Autodesk Inventor part; units mm, degrees
ref_plane "YZ Plane" through (0, 0, 0) normal (1, 0, 0) x (0, 1, 0)
ref_plane "XZ Plane" through (0, 0, 0) normal (0, 1, 0) x (-1, 0, 0)
ref_plane "XY Plane" through (0, 0, 0) normal (0, 0, 1) x (1, 0, 0)
sketch "Sketch1" plane through (0, 0, 0) normal (0, 0, 1) x (1, 0, 0)
  line L0 (5.5, 34.5) -> (27, 34.5)
  line L1 (1.5, 2.5) -> (27, 2.5)
  line L2 (27, 2.5) -> (27, 34.5)
  line L3 (27, 34.5) -> (5.5, 34.5)
  line L4 (1.5, 35.5) -> (1.5, 2.5)
  line L5 (1.5, 76.5) -> (5.5, 76.5)
  line L6 (1.5, 2.5) -> (5.5, 2.5)
  line L7 (5.5, 34.5) -> (5.5, 76.5)
  line L8 (5.5, 76.5) -> (1.5, 76.5)
  line L9 (1.5, 76.5) -> (1.5, 2.5)
  point P0 (0, 0)
  dimension "d0" = 32
  dimension "d2" = 21.5
  dimension "d3" = 42
  dimension "d17" = 4
extrude "Extrusion1" add sketch "Sketch1" along normal blind 1.5
sketch "Sketch2" plane through (0, 0, 0) normal (0, 0, -1) x (-1, 0, 0)
  line L0 (-27, 2.5) -> (-27, 34.5)
  line L1 (-27, 34.5) -> (-5.5, 34.5)
  line L2 (-5.5, 34.5) -> (-5.5, 26.5)
  line L3 (-5.5, 26.5) -> (-27, 26.5)
  line L4 (-27, 26.5) -> (-27, 34.5)
  line L5 (-1.5, 2.5) -> (-27, 2.5)
  line L6 (-27, 2.5) -> (-5.5, 2.5)
  line L7 (-5.5, 2.5) -> (-5.5, 10.5)
  line L8 (-5.5, 10.5) -> (-27, 10.5)
  line L9 (-27, 10.5) -> (-27, 2.5)
  point P0 (0, 0)
  point P1 (-27, 10.5)
  point P2 (-27, 26.5)
  dimension "d6" = 16
extrude "Extrusion2" add sketch "Sketch2" along normal blind 4.5
sketch "Sketch3" plane through (0, 0, 1.5) normal (0, 0, 1) x (1, 0, 0)
  circle A0 centre (8.5, 32.5) radius 1
  circle A1 centre (18.5, 4.5) radius 1
  line L0 (27, 2.5) -> (27, 34.5)
  line L1 (1.5, 2.5) -> (27, 2.5)
  line L2 (27, 34.5) -> (5.5, 34.5)
  point P0 (0, 0)
  dimension "d9" = 2
  dimension "d10" = 2
  dimension "d11" = 18.5
  dimension "d12" = 8.5
  dimension "d13" = 2
  dimension "d14" = 2
extrude "Extrusion3" cut sketch "Sketch3" against normal through all
chamfer "Chamfer1" distance 1.5 angle 45 2 edges at (7.5, 32.5, 1.5) (17.5, 4.5, 1.5)
properties part number "servoholder"
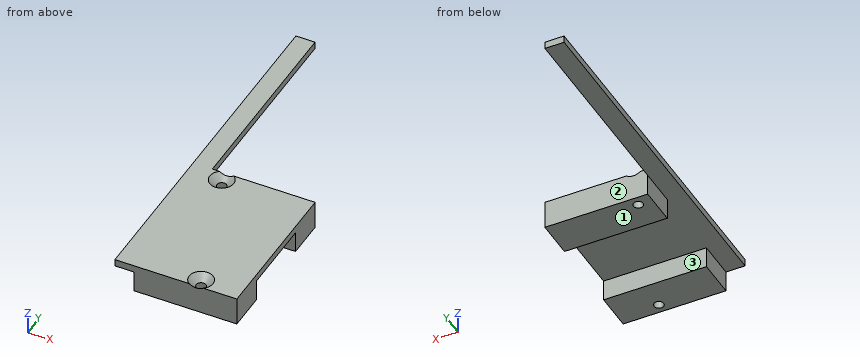
Part model, mm, in its own coordinate system. Face numbers are marked on the shaded views. A direction names the side the tool comes from. Coordinates: 2 decimals unless noted, no trailing zeros. Order: outer loops, then holes, each group sorted by start corner. A loop starts at its lowest first (then second) coordinate and runs counter-clockwise, first axis right, second up.
(1) Slice it at B-B, the plane y = 32.5. Write the cut outline in (x, z), and give its area (3 significant figures).
Check sheet entries:
outline: (1.5, 0) - (5.5, 0) - (5.5, -4.5) - (7.5, -4.5) - (7.5, 0) - (6, 1.5) - (1.5, 1.5) - close; (9.5, -4.5) - (27, -4.5) - (27, 1.5) - (11, 1.5) - (9.5, 0) - close
area: 121 mm2
(2) Slice it at D-D, the plane x = 23.75. Write the cut outline in (y, z), and give its area (3 significant figures).
Check sheet entries:
outline: (2.5, -4.5) - (10.5, -4.5) - (10.5, 0) - (26.5, 0) - (26.5, -4.5) - (34.5, -4.5) - (34.5, 1.5) - (2.5, 1.5) - close
area: 120 mm2
(3) Pin check, flat tips, straight feed: pin 1 Ø1.6 at (y, z) = (65.5, 0.5) entering from +X; pin 2 Ø2 at (x, z) = (15, -0.5) entering from +Y; pin 3 Ø1.6 at (x, y) = (8.5, 32.5) entering from -Z; pin 4 Ø1.3 at (y, z) = (31, -1) entering from -X. Stop position of each tip, or through.
Check sheet entries:
pin 1: stops at x = 5.5
pin 2: stops at y = 34.5
pin 3: passes through
pin 4: stops at x = 5.5
(4) Probe L1, parallel to Y at x = 18.5, z = -3.05; L2, parallel to Y at x = 8.5, z = -3.35; L3, parallel to Y at x = 20.5, z = -3. List the from-to ranges inside material, lowest first.
Check sheet entries:
L1: y = 2.5 to 3.5, 5.5 to 10.5, 26.5 to 34.5
L2: y = 2.5 to 10.5, 26.5 to 31.5, 33.5 to 34.5
L3: y = 2.5 to 10.5, 26.5 to 34.5
(5) Slice it at C-C, the plane x = 18.5. Write the cut outline in (y, z), and give its area (3 significant figures).
Check sheet entries:
outline: (2.5, -4.5) - (3.5, -4.5) - (3.5, 0) - (2.5, 1) - close; (5.5, -4.5) - (10.5, -4.5) - (10.5, 0) - (26.5, 0) - (26.5, -4.5) - (34.5, -4.5) - (34.5, 1.5) - (7, 1.5) - (5.5, 0) - close
area: 106 mm2
(6) Slice it at A-A, the plane z = -2.7. Write the cut outline in (x, y), and give its area (3 significant figures).
Check sheet entries:
outline: (5.5, 2.5) - (27, 2.5) - (27, 10.5) - (5.5, 10.5) - close; (5.5, 26.5) - (27, 26.5) - (27, 34.5) - (5.5, 34.5) - close; hole circle Ø2 at (8.5, 32.5); hole circle Ø2 at (18.5, 4.5)
area: 338 mm2
(7) Tool access for the marked faces 1, 2 and 3: list every direction of +Z, -Z, +X, -X, +Y, -Y with a clear straight run to the whole face (end or side of a thin tool).
Check sheet entries:
face 1: -Z, +X, -X, +Y, -Y
face 2: +Z, -Z, +X, +Y
face 3: -Z, +X, -X
